```python
from build123d import *

# Parameters (mm, degrees)
BOSS_EXTRUDE1_DEPTH = 8
CHAMFER1_SIZE       = 2
SKETCH2_R           = 1.5
CUT_EXTRUDE1_DEPTH  = 25.397745798
FILLET1_R           = 4
SKETCH3_R           = 2
CUT_EXTRUDE2_DEPTH  = 28.753378173
CHAMFER2_SIZE       = 2


with BuildPart() as part:
    # Sketch1 → Boss-Extrude1 (new body)
    with BuildSketch(Plane(origin=(0, 0, 0), x_dir=(1, 0, 0), z_dir=(0, 1, 0))):
        with BuildLine():
            Line((10, 20), (-10, 20))
            Line((-10, 20), (-10, 5))
            Line((-10, 5), (-17.5, 5))
            Line((-17.5, 5), (-17.5, 0))
            Line((-17.5, 0), (-3, 0))
            ThreePointArc((-3, 0), (0, 3), (3, 0))
            Line((3, 0), (17.5, 0))
            Line((17.5, 0), (17.5, 5))
            Line((17.5, 5), (10, 5))
            Line((10, 5), (10, 20))
        make_face()
    extrude(amount=BOSS_EXTRUDE1_DEPTH)

    # Chamfer1
    chamfer1_edges = [part.edges().sort_by_distance(p)[0] for p in [
        (-10, 4, -5),
        (10, 4, -5),
    ]]
    chamfer(chamfer1_edges, length=CHAMFER1_SIZE)

    # Sketch2 → Cut-Extrude1 (cut, through all)
    with BuildSketch(Plane(origin=(0, 0, -5), x_dir=(-1, 0, 0), z_dir=(0, 0, -1))):
        with Locations((-15, 4)):
            Circle(SKETCH2_R)
        with Locations((15, 4)):
            Circle(SKETCH2_R)
    extrude(amount=-CUT_EXTRUDE1_DEPTH, mode=Mode.SUBTRACT)

    # Fillet1
    fillet1_edges = [part.edges().sort_by_distance(p)[0] for p in [
        (17.5, 8, -2.5),
        (-17.5, 8, -2.5),
        (17.5, 0, -2.5),
        (-17.5, 0, -2.5),
    ]]
    fillet(fillet1_edges, radius=FILLET1_R - 0.0001)  # a hair under: the kernel refuses the full size

    # Sketch3 → Cut-Extrude2 (cut, through all)
    with BuildSketch(Plane(origin=(0, 8, 0), x_dir=(1, 0, 0), z_dir=(0, 1, 0))):
        with Locations(Location((-6.122934918, 14.78207252, 0), (0, 0, 270))):
            Circle(SKETCH3_R)
        with Locations(Location((6.122934918, 14.78207252, 0), (0, 0, 270))):
            Circle(SKETCH3_R)
    extrude(amount=-CUT_EXTRUDE2_DEPTH, mode=Mode.SUBTRACT)

    # Chamfer2
    chamfer2_edges = [part.edges().sort_by_distance(p)[0] for p in [
        (-10, 4, -20),
        (10, 4, -20),
    ]]
    chamfer(chamfer2_edges, length=CHAMFER2_SIZE)


solid = part.part
```
Check sheet for the modelled part. Datum: model origin and axes. Units: mm. A direction names the side the tool comes from. Coordinates: 2 decimals unless noted, no trailing zeros. Write each loop counter-clockwise with the first axis right and the second up, starting at its lowest first coordinate (ties: lowest second). Pieces come first, ordered by that corner, then holes. Notation, with made-up numbers: M 88.5,-8 L 107.5,-8 A32 ccw 107.5,28 Z; hole C 59.25,-35 d7. An arc over 180 degrees is marked long. Write item = value, one per line. Start each with the question number.
1. Mould release check, pull along X, two halves, no side actions. Record for faces 4 (the cylindrical face through (-16.297, 1.141, -2.465)), 5 (the cylindrical face through (16.5, 4.07, -2.54)), 6 (the flat face through (0, 0, -10)): pulls with the +X half, pulls with the -X half, needs draft (parallel to the pull), parting line crosses it, or undercut.
2. Thickness scan on probe 1 along X at (y, z) = (3, -4.25); probe 2 along X at (y, z) = (1.5, -13.5); probe 3 along X at (y, z) = (1.5, -12.5). Record the ranges inside material, lowest first.
3. Sectioned sample at C-C (z = -14.25). Record the cut outline in (x, y) (3 decimals).
4. Sectioned sample at B-B (y = 3). Record the cut outline in (x, z), then the cut area to 3 significant figures.
5. Tool access check on faces 1 (the flat face through (-13, 4, -5)), 2 (the flat face through (10, 4, -12)), 3 (the cylindrical face through (6.724, 4.056, -12.874)). Record the directions out of +Z, -Z, +X, -X, +Y, -Y that give a thin tool (end or side, any length) a straight path to the whole face; none if there is none.
6. Sectioned sample at D-D (z = -17.5). Record the cut outline in (x, y), then the cut area to 3 significant figures.
7. Sectioned sample at A-A (x = 15). Record the cut outline in (y, z).
8. Go/stop test with flat-tipped pins: pin 1 (3 mm diameter, centred on x = 15.5, y = 3.5, fed in from -Z); pin 2 (2.5 mm diameter, centred on y = 5.5, z = -14.5, fed in from +X); pin 3 (1.5 mm diameter, centred on y = 6.5, z = -10.5, fed in from -X). Record where each tip stops, or that it passes through.
The answers:
q1.face_4 = pulls with the -X half
q1.face_5 = undercut
q1.face_6 = needs draft
q2.probe_1 = -17.37 to -16.12, -13.88 to 13.88, 16.12 to 17.37
q2.probe_2 = -10 to -7.66, -4.59 to 4.59, 7.66 to 10
q2.probe_3 = -10 to 10
q3.outline = M -10,0 L -8.051,0 L -8.051,8 L -10,8 Z; M -4.195,0 L 4.195,0 L 4.195,8 L -4.195,8 Z; M 8.051,0 L 10,0 L 10,8 L 8.051,8 Z
q4.outline = M -17.37,-5 L -16.12,-5 L -16.12,0 L -17.37,0 Z; M -13.88,-5 L -12,-5 L -10,-7 L -10,-18 L -8,-20 L 8,-20 L 10,-18 L 10,-7 L 12,-5 L 13.88,-5 L 13.88,0 L 3,0 A3 cw -3,0 L -13.88,0 Z; M 16.12,-5 L 17.37,-5 L 17.37,0 L 16.12,0 Z; hole C -6.12,-14.78 d4; hole C 6.12,-14.78 d4
q4.area = 412 mm²
q5.face_1 = -Z, -X, +Y, -Y
q5.face_2 = -Z, +X, +Y, -Y
q5.face_3 = +Y, -Y
q6.outline = M -10,0 L 10,0 L 10,8 L -10,8 Z
q6.area = 160 mm²
q7.outline = M 0.29,-5 L 2.5,-5 L 2.5,0 L 0.29,0 Z; M 5.5,-5 L 7.71,-5 L 7.71,0 L 5.5,0 Z
q8.pin_1 = -5
q8.pin_2 = 10
q8.pin_3 = -10
